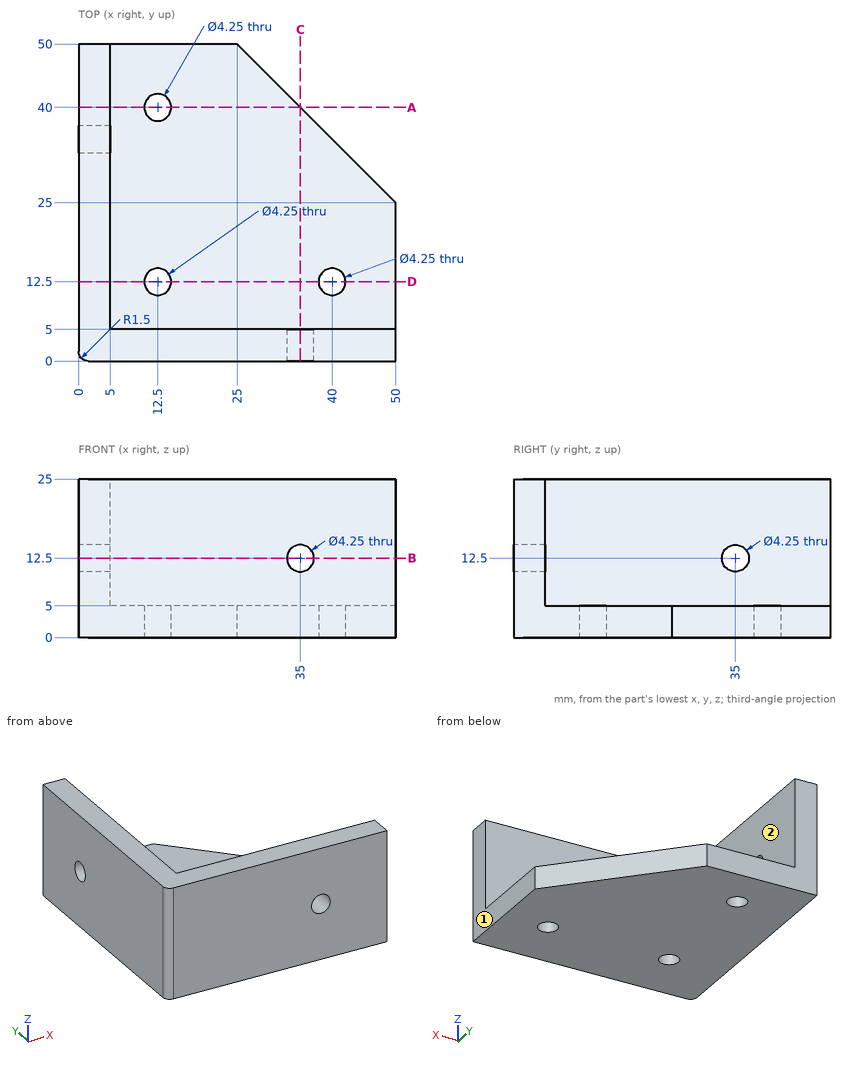
Could you check a few things on this drawing? It's one solid part, dimensions in mm from its lowest x, y, z. A direction names the side the tool comes from. Give positions to 0.01 mm unless a question says otherwise; leave off trailing zeros. Order: outer loops, then holes, each group sorted by start corner. A loop starts at its lowest first (then second) coordinate and runs counter-clockwise, first axis right, second up. Notation, with made-up numbers: (71.25, -24.5) - (89.25, -24.5) arc R30 ccw to (89.25, 0.5) - close; hole circle Ø4 at (-24.75, -21). An arc over 180 degrees is marked (long way). One line per question, with ' | ' between items. Start each with the question number.
Item 1: For the marked faces 1 and 2, which set-ups out of +Z, -Z, +X, -X, +Y, -Y let a thin tool reach every point of the face, with its end or its side?
Item 2: I need wall thicknesses on probe 1 along Z at (x, y) = (37, 21). Which ranges of the line are inside material? Lowest first, please. Write a range as [from, to].
Item 3: I want a section at B-B on z = 12.5. Write out the boundary of the cut face in (x, y) (3 decimals).
Item 4: I want a section at C-C on x = 35. Write out the boundary of the cut face in (y, z) (3 decimals).
Item 5: I'm going to push flat-ended pins straight in: pin 1 Ø3 at (x, y) = (35.5, 12.5) entering from +Z; pin 2 Ø8 at (x, z) = (9.5, 21) entering from +Y; pin 3 Ø10 at (y, z) = (35.5, 18.5) entering from +X. Where does each tip first touch, or does it pass through?
Item 6: I want a section at A-A on y = 40. Write out the boundary of the cut face in (x, z) (3 decimals), then the cut area to 3 significant figures.
Item 7: I want a section at D-D on y = 12.5. Write out the boundary of the cut face in (x, z) (3 decimals), then the cut area to 4 significant figures.
Verdict:
1) face 1: +Z, -Z, +X, +Y, -Y | face 2: +Z, +X, +Y
2) probe 1: [0, 5]
3) outline: (0, 1.5) arc R1.5 ccw to (1.5, 0) - (32.875, 0) - (32.875, 5) - (5, 5) - (5, 32.875) - (0, 32.875) - close; (0, 37.125) - (5, 37.125) - (5, 50) - (0, 50) - close; (37.125, 0) - (50, 0) - (50, 5) - (37.125, 5) - close
4) outline: (0, 0) - (40, 0) - (40, 5) - (5, 5) - (5, 10.375) - (0, 10.375) - close; (0, 14.625) - (5, 14.625) - (5, 25) - (0, 25) - close
5) pin 1: z = 5 | pin 2: y = 5 | pin 3: x = 5
6) outline: (0, 0) - (10.375, 0) - (10.375, 5) - (5, 5) - (5, 25) - (0, 25) - close; (14.625, 0) - (35, 0) - (35, 5) - (14.625, 5) - close | area: 254 mm^2
7) outline: (0, 0) - (10.375, 0) - (10.375, 5) - (5, 5) - (5, 25) - (0, 25) - close; (14.625, 0) - (37.875, 0) - (37.875, 5) - (14.625, 5) - close; (42.125, 0) - (50, 0) - (50, 5) - (42.125, 5) - close | area: 307.5 mm^2
